Check sheet for the modelled part. Datum: model origin and axes. Units: mm. A direction names the side the tool comes from. Give positions to 0.01 mm unless a question says otherwise; leave off trailing zeros. Order: outer loops, then holes, each group sorted by start corner. A loop starts at its lowest first (then second) coordinate and runs counter-clockwise, first axis right, second up.
Item 1: Sectioned sample at C-C on x = -9.75. Record the boundary of the cut face in (y, z), and give its area (3 significant figures).
Item 2: Access from +Z, -Z, +X, -X, +Y, -Y to the whole of each face (thin tool, end or side, straight path). Record for faces 4 (the flat face through (4.748, 6.574, 6.927)), 5 (the flat face through (1.541, 6.574, -8.256)), 6 (the flat face through (-6.927, 6.574, 4.748)), 7 (the flat face through (-2.6, 3, -8.2)).
Item 3: Sectioned sample at B-B on z = -4.25. Record the boundary of the cut face in (x, y), and give its area (3 significant figures).
Item 4: Gauge pin test, flat ends, axial feed: P1, Ø10, axis at y = 5.5, z = 6.5, coming from the +X side; P2, Ø1, axis at y = 9, z = -5, coming from the -X side; P3, Ø1, axis at y = 7, z = -10, coming from the -X side; P4, Ø2, axis at y = 18, z = -7.5, coming from the +X side. Record the tip position at first contact, or that the pin passes through.
Item 5: Release check for a two-part mould opening along Z. For faces 1 (the flat face through (2.6, 10.25, 8.2)), 2 (the flat face through (1.735, 6.574, 8.217)), 3 (the cylindrical face through (-1.19, 12.8, 5.37)) record: released by +Z, released by -Z, zero draft, split by the parting line, or undercut.
Item 6: Sectioned sample at A-A on x = 2. Record the boundary of the cut face in (y, z), and give its area (3 significant figures).
Item 7: Material ranges on line 1 along Y through (x, z) = (7, 6); line 2 along Z through (x, y) = (0, 12.25), recorded low to high.
Autodesk Inventor part; units mm, degrees
ref_plane "YZ Plane" through (0, 0, 0) normal (1, 0, 0) x (0, 1, 0)
ref_plane "XZ Plane" through (0, 0, 0) normal (0, 1, 0) x (-1, 0, 0)
ref_plane "XY Plane" through (0, 0, 0) normal (0, 0, 1) x (1, 0, 0)
sketch "Szkic1" plane through (0, 0, 0) normal (0, 1, 0) x (-1, 0, 0)
  circle A0 centre (0, 0) radius 12.5
  dimension "d0" = 25
extrude "Wyciągnięcie proste1" add sketch "Szkic1" along normal blind 3
sketch "Szkic7" plane through (0, 3, 0) normal (0, 1, 0) x (1, 0, 0)
  line L0 (6, 6.109) -> (7.8811, 3.3479)
  line L1 (7.8811, 3.3479) -> (8.5624, 0.0771)
  line L2 (8.5624, 0.0771) -> (7.9401, -3.2055)
  line L3 (7.9401, -3.2055) -> (6.109, -6)
  line L4 (6.109, -6) -> (3.3479, -7.8811)
  line L5 (3.3479, -7.8811) -> (0.0771, -8.5624)
  line L6 (0.0771, -8.5624) -> (-3.2055, -7.9401)
  line L7 (-3.2055, -7.9401) -> (-6, -6.109)
  line L8 (-6, -6.109) -> (-7.8811, -3.3479)
  line L9 (-7.8811, -3.3479) -> (-8.5624, -0.0771)
  line L10 (-8.5624, -0.0771) -> (-7.9401, 3.2055)
  line L11 (-7.9401, 3.2055) -> (-6.109, 6)
  line L12 (-6.109, 6) -> (-3.3479, 7.8811)
  line L13 (-3.3479, 7.8811) -> (-0.0771, 8.5624)
  line L14 (-0.0771, 8.5624) -> (3.2055, 7.9401)
  line L15 (3.2055, 7.9401) -> (6, 6.109)
  point P0 (0, 0)
  point P1 (0, 0)
extrude "Wyciągnięcie proste6" add sketch "Szkic7" along normal blind 7.25
sketch "Szkic8" plane through (0, 10.25, 0) normal (0, 1, 0) x (1, 0, 0)
  circle A0 centre (0, 0) radius 12.5
extrude "Wyciągnięcie proste7" add sketch "Szkic8" along normal blind 15
sketch "Szkic9" plane through (0, 25.25, 0) normal (0, 1, 0) x (1, 0, 0)
  circle A0 centre (0, 0) radius 5.5016
extrude "Wyciągnięcie proste8" cut sketch "Szkic9" against normal blind 30
sketch "Szkic10" plane through (0, 25.25, 0) normal (0, 1, 0) x (1, 0, 0)
  point P0 (0, 0)
properties part number "spool_long"
Report:
1. outline: (0, -7.82) - (3, -7.82) - (3, 7.82) - (0, 7.82) - close; (10.25, -7.82) - (25.25, -7.82) - (25.25, 7.82) - (10.25, 7.82) - close
1. area: 282 mm2
2. face 4: +Z, +X
2. face 5: -Z, +X
2. face 6: +Z, -X
2. face 7: none
3. outline: (-11.76, 0) - (-3.49, 0) - (-3.49, 25.25) - (-11.76, 25.25) - (-11.76, 10.25) - (-7.26, 10.25) - (-7.26, 3) - (-11.76, 3) - close; (3.49, 0) - (11.76, 0) - (11.76, 3) - (7.27, 3) - (7.27, 10.25) - (11.76, 10.25) - (11.76, 25.25) - (3.49, 25.25) - close
3. area: 352 mm2
4. P1: stops at x = 12.31
4. P2: stops at x = -7.09
4. P3: passes through
4. P4: stops at x = 10.68
5. face 1: zero draft
5. face 2: released by +Z
5. face 3: undercut
6. outline: (0, -12.34) - (3, -12.34) - (3, -8.17) - (10.25, -8.17) - (10.25, -12.34) - (25.25, -12.34) - (25.25, -5.13) - (0, -5.13) - close; (0, 5.13) - (25.25, 5.13) - (25.25, 12.34) - (10.25, 12.34) - (10.25, 8.16) - (3, 8.16) - (3, 12.34) - (0, 12.34) - close
6. area: 304 mm2
7. line 1: y = 0 to 3, 10.25 to 25.25
7. line 2: z = -12.5 to -5.5, 5.5 to 12.5
